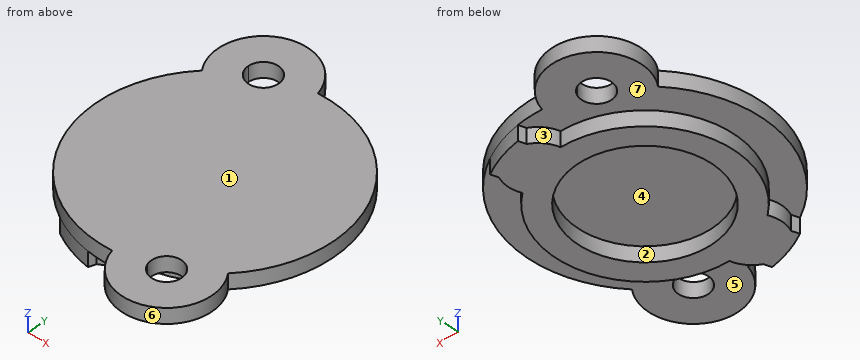
from build123d import *
from build123d.topology import SkipClean

# Parameters (mm, degrees)
SKETCH1_R           = 7.85
BOSS_EXTRUDE1_DEPTH = 1
BOSS_EXTRUDE2_START = 1
SKETCH3_R           = 6
SKETCH3_R_2         = 4.5
BOSS_EXTRUDE2_DEPTH = 1
BOSS_EXTRUDE3_DEPTH = 1
SKETCH2_3_R         = 1
CUT_EXTRUDE1_DEPTH  = 2
SKETCH2_4_R         = 1
CUT_EXTRUDE2_DEPTH  = 3


with BuildPart() as part:
    # Sketch1 → Boss-Extrude1 (new body)
    with BuildSketch(Plane.XY):
        Circle(SKETCH1_R)
    extrude(amount=BOSS_EXTRUDE1_DEPTH)

    # Sketch3 → Boss-Extrude2 (add)
    # profile 1 of 3: a face of its own
    with SkipClean():  # the faces are left unmerged after this step: merging them gives an invalid solid
        with BuildSketch(Plane(origin=(0, 0, 0), x_dir=(-1, 0, 0), z_dir=(0, 0, -1)).offset(BOSS_EXTRUDE2_START)):
            Circle(SKETCH3_R)
            Circle(SKETCH3_R_2, mode=Mode.SUBTRACT)
        # profile 2 of 3: a face of its own
        with BuildSketch(Plane(origin=(0, 0, 0), x_dir=(-1, 0, 0), z_dir=(0, 0, -1)).offset(BOSS_EXTRUDE2_START)):
            with BuildLine():
                ThreePointArc((3.757317387, -4.677880508), (1.992185075, -5.659611173), (0.001300165, -5.999999859))
                ThreePointArc((0.001300165, -5.999999859), (0.375700996, -6.761308528), (1.032012818, -7.298915878))
                Line((1.032012818, -7.298915878), (1.193852248, -7.758686539))
                ThreePointArc((1.193852248, -7.758686539), (2.606442139, -7.404657951), (3.929330982, -6.795797086))
                Line((3.929330982, -6.795797086), (3.767491551, -6.336026426))
                ThreePointArc((3.767491551, -6.336026426), (3.9423428, -5.505849389), (3.757317387, -4.677880508))
            make_face()
        # profile 3 of 3: a face of its own
        with BuildSketch(Plane(origin=(0, 0, 0), x_dir=(-1, 0, 0), z_dir=(0, 0, -1)).offset(BOSS_EXTRUDE2_START)):
            with BuildLine():
                Line((-3.929330982, 6.795797086), (-3.767491551, 6.336026426))
                ThreePointArc((-3.767491551, 6.336026426), (-3.9423428, 5.505849389), (-3.757317387, 4.677880508))
                ThreePointArc((-3.757317387, 4.677880508), (-1.992185075, 5.659611173), (-0.001300165, 5.999999859))
                ThreePointArc((-0.001300165, 5.999999859), (-0.375700996, 6.761308528), (-1.032012818, 7.298915878))
                Line((-1.032012818, 7.298915878), (-1.193852248, 7.758686539))
                ThreePointArc((-1.193852248, 7.758686539), (-2.606442139, 7.404657951), (-3.929330982, 6.795797086))
            make_face()
        extrude(amount=-BOSS_EXTRUDE2_DEPTH)

    # Sketch2 → Boss-Extrude3 (add)
    with BuildSketch(Plane(origin=(0, 0, 0), x_dir=(-1, 0, 0), z_dir=(0, 0, -1))):
        with BuildLine():
            ThreePointArc((-4.265263368, -6.590146311), (-5.074768612, -5.989092046), (-5.800557161, -5.289237811))
            ThreePointArc((-5.800557161, -5.289237811), (-4.68948187, -9.784235269), (-0.489616971, -7.834716027))
            ThreePointArc((-0.489616971, -7.834716027), (-1.489786667, -7.707336485), (-2.46537987, -7.452811691))
            ThreePointArc((-2.46537987, -7.452811691), (-3.825061249, -7.980689597), (-4.265263368, -6.590146311))
        make_face()
        with BuildLine():
            ThreePointArc((2.46537987, 7.452811691), (3.583283252, 8.060617089), (4.392850938, 7.078916761))
            ThreePointArc((4.392850938, 7.078916761), (4.360428436, 6.826342445), (4.265263368, 6.590146311))
            ThreePointArc((4.265263368, 6.590146311), (5.074768612, 5.989092046), (5.800557161, 5.289237811))
            ThreePointArc((5.800557161, 5.289237811), (4.68948187, 9.784235269), (0.489616971, 7.834716027))
            ThreePointArc((0.489616971, 7.834716027), (1.489786667, 7.707336485), (2.46537987, 7.452811691))
        make_face()
    extrude(amount=-BOSS_EXTRUDE3_DEPTH)

    # Sketch2<3> → Cut-Extrude1 (cut)
    with BuildSketch(Plane(origin=(0, 0, 0), x_dir=(-1, 0, 0), z_dir=(0, 0, -1))):
        with Locations((3.392850938, 7.078916761)):
            Circle(SKETCH2_3_R)
    extrude(amount=-CUT_EXTRUDE1_DEPTH, mode=Mode.SUBTRACT)

    # Sketch2<4> → Cut-Extrude2 (cut)
    with BuildSketch(Plane(origin=(0, 0, 0), x_dir=(-1, 0, 0), z_dir=(0, 0, -1))):
        with Locations((-3.392850938, -7.078916761)):
            Circle(SKETCH2_4_R)
    extrude(amount=-CUT_EXTRUDE2_DEPTH, mode=Mode.SUBTRACT)


solid = part.part
The model under review builds one solid part; all positions refer to its coordinate system, in mm. Face numbers are marked on the shaded views. A direction names the side the tool comes from. Round coordinates to 2 decimals unless told otherwise and drop trailing zeros. Write each loop counter-clockwise with the first axis right and the second up, starting at its lowest first coordinate (ties: lowest second). Pieces come first, ordered by that corner, then holes. Notation, with made-up numbers: (15.25, 58.25) -> (67.25, 58.25) arc R15 ccw to (67.25, 87.25) -> close; hole circle Ø10 at (30, 26.25). An arc over 180 degrees is marked (long way). Answer as a JSON object with one key per item and string values.
1. The part is to be moulded in two halves that separate along X. For the marked faces 1, 2 and 3, say which applies: pulls with the +X half, pulls with the -X half, needs draft (parallel to the pull), parting line crosses it, or undercut.
Results found:
{"face 1": "needs draft", "face 2": "undercut", "face 3": "pulls with the -X half"}
2. To check wall thickness, follow line 1 along Z through (x, y) = (-4.5, 9); line 2 along Y through (x, z) = (6, 0.8); line 3 along Y through (x, z) = (0, 0.15). State the ranges of each line that lie inside material, in increasing order.
Results found:
{"line 1": "z = 0 to 1", "line 2": "y = -8.56 to -5.59, -5.06 to 5.06", "line 3": "y = -7.85 to 7.85"}
3. We need section C-C on x = 5.5. State the section outline as (y, z) points, and give its area (3 significant figures).
Results found:
{"outline": "(-9.21, 0) -> (-2.4, 0) -> (-2.4, -1) -> (2.4, -1) -> (2.4, 0) -> (5.6, 0) -> (5.6, 1) -> (-9.21, 1) -> close", "area": "19.6 mm^2"}
4. Clearance check with a flat-ended pin moving along its axis: pin 1 (7 mm diameter, centred on x = 0, y = 0, fed in from -Z). State where the tip first meets the part, or that it passes through.
Results found:
{"pin 1": "stops at z = 0"}
5. We need section A-A on z = -0.35. State the section outline as (x, y) points, and give its area (3 significant figures).
Results found:
{"outline": "(-3.93, -6.8) arc R7.85 ccw to (-1.19, -7.76) -> (-1.03, -7.3) arc R2 ccw to (0, -6) arc R6 ccw to (3.76, 4.68) arc R2 ccw to (3.77, 6.34) -> (3.93, 6.8) arc R7.85 ccw to (1.19, 7.76) -> (1.03, 7.3) arc R2 ccw to (0, 6) arc R6 ccw to (-3.76, -4.68) arc R2 ccw to (-3.77, -6.34) -> close; hole circle Ø9 at (0, 0)", "area": "62.6 mm^2"}
6. We need section D-D on y = -3. State the section outline as (x, z) points.
Results found:
{"outline": "(-7.25, 0) -> (-5.2, 0) -> (-5.2, -1) -> (-3.35, -1) -> (-3.35, 0) -> (3.35, 0) -> (3.35, -1) -> (5.2, -1) -> (5.2, 0) -> (7.25, 0) -> (7.25, 1) -> (-7.25, 1) -> close"}
7. We need section B-B on y = 0. State the section outline as (x, z) points, and give its area (3 significant figures).
Results found:
{"outline": "(-7.85, 0) -> (-6, 0) -> (-6, -1) -> (-4.5, -1) -> (-4.5, 0) -> (4.5, 0) -> (4.5, -1) -> (6, -1) -> (6, 0) -> (7.85, 0) -> (7.85, 1) -> (-7.85, 1) -> close", "area": "18.7 mm^2"}
8. Machinability: for the marked faces 4, 5, 6 and 7, which of the approach directions +Z, -Z, +X, -X, +Y, -Y give a long, thin tool a straight path to every point of the face, cutting with its end or side? Answer none if there is none.
Results found:
{"face 4": "-Z", "face 5": "-Z, +X", "face 6": "+Z, -Z", "face 7": "-Z, -X"}
